Autodesk Inventor part; units mm, degrees
ref_plane "YZ Plane" through (0, 0, 0) normal (1, 0, 0) x (0, 1, 0)
ref_plane "XZ Plane" through (0, 0, 0) normal (0, 1, 0) x (-1, 0, 0)
ref_plane "XY Plane" through (0, 0, 0) normal (0, 0, 1) x (1, 0, 0)
sketch "Sketch1" plane through (0, 0, 0) normal (1, 0, 0) x (0, 1, 0)
  line L0 (0, 0) -> (4.7625, 0)
  line L1 (4.7625, 0) -> (4.7625, -168.8592)
  line L2 (4.7625, -168.8592) -> (0, -168.8592)
  line L3 (0, -168.8592) -> (0, 0)
  dimension "d1" = 4.7625
  dimension "d2" = 168.8592
extrude "Extrusion1" add sketch "Sketch1" along normal blind 0.7937
sketch "Sketch2" plane through (0, 0, -168.8592) normal (0, 0, -1) x (-1, 0, 0)
  line L0 (-0.7937, 0) -> (-0.7937, 4.7625)
  line L1 (-0.7937, 0) -> (36.0362, 0)
  line L2 (36.0362, 0) -> (36.0362, 4.7625)
  line L3 (36.0362, 4.7625) -> (-0.7937, 4.7625)
  line L4 (-0.7937, 4.7625) -> (-0.7937, 0)
  point P0 (0, 0)
  dimension "d5" = 36.83
  dimension "d6" = 4.7625
extrude "Extrusion2" add sketch "Sketch2" against normal blind 0.7937
sketch "Sketch3" plane through (-36.0362, 0, -168.8592) normal (-1, 0, 0) x (0, 0, 1)
  line L0 (168.8592, 4.7625) -> (168.8592, 0)
  line L1 (0, 0) -> (168.8592, 0)
  line L2 (168.8592, 0) -> (168.8592, 4.7625)
  line L3 (168.8592, 4.7625) -> (0, 4.7625)
  line L4 (0, 4.7625) -> (0, 0)
extrude "Extrusion3" add sketch "Sketch3" against normal blind 0.7937
sketch "Sketch4" plane through (-36.0362, 0, 0) normal (0, 0, 1) x (1, 0, 0)
  line L0 (0, 0) -> (0, 4.7625)
  line L1 (36.0362, 4.7625) -> (36.83, 4.7625)
  line L2 (0, 0) -> (36.83, 0)
  line L3 (36.83, 0) -> (36.83, 4.7625)
  line L4 (36.83, 4.7625) -> (0, 4.7625)
  line L5 (0, 4.7625) -> (0, 0)
  point P0 (36.0362, 0)
extrude "Extrusion4" add sketch "Sketch4" against normal blind 0.7937
sketch "Sketch7" plane through (-36.0362, 0, 0) normal (0, 0, 1) x (1, 0, 0)
  circle A0 centre (18.415, 2.3812) radius 2.2098
extrude "Extrusion5" cut sketch "Sketch7" against normal blind 0.7937
sketch "Sketch6" plane through (0.7937, 0, -168.8592) normal (0, 0, -1) x (-1, 0, 0)
  circle A0 centre (18.415, 2.3812) radius 2.2098
extrude "Extrusion6" cut sketch "Sketch6" against normal blind 0.7937
properties part number "Back rubber bands"
The listing builds one solid part. Answer for the finished solid, in the listing's coordinates (mm). A direction names the side the tool comes from. Give positions to 0.01 mm unless a question says otherwise; leave off trailing zeros. Write each loop counter-clockwise with the first axis right and the second up, starting at its lowest first coordinate (ties: lowest second). Pieces come first, ordered by that corner, then holes. Notation, with made-up numbers: (31.5, 23.25) -> (36.5, 23.25) arc R25 ccw to (36.5, 50.25) -> close; hole circle Ø4 at (89, 39.5). An arc over 180 degrees is marked (long way). Write item = value, one per line. Start each with the question number.
1) The part is cut by section B-B, the plane x = -13. Determine the outline of the cut face in (y, z).
2) Which of the six approach directions +Z, -Z, +X, -X, +Y, -Y give full straight-line access (tool end or side, diameter ignored) to faces 5 (the face through (0, 2, -83)), 6 (the face through (-35.4, 4.762, -84))?
3) Determine the mould class of faces 1 (the face through (-14, 2, 0)), 2 (the face through (0.794, 2, -84)), 3 (the face through (-36.036, 2, -86)), 4 (the face through (-19.83, 2.48, -0.39)) for opening direction X: +X half, -X half, draft (parallel to the pull), parting line (faces both ways), or undercut.
4) Straight lines are drawn through the part: line 1 along X through (y, z) = (4, -52.5); line 2 along Z through (x, y) = (-5, 3.75). For each, find the intervals that lie inside material, in ascending order.
5) The part is cut by section A-A, the plane z = -86. Determine the outline of the cut face in (x, y).
Solutions:
q1.outline = (0, -168.86) -> (4.76, -168.86) -> (4.76, -168.07) -> (0, -168.07) -> close; (0, -0.79) -> (4.76, -0.79) -> (4.76, 0) -> (0, 0) -> close
q2.face_5 = +Y, -Y
q2.face_6 = +Z, -Z, +X, -X, +Y
q3.face_1 = draft
q3.face_2 = +X half
q3.face_3 = -X half
q3.face_4 = undercut
q4.line_1 = -36.04 to -35.24, 0 to 0.79
q4.line_2 = -168.86 to -168.07, -0.79 to 0
q5.outline = (-36.04, 0) -> (-35.24, 0) -> (-35.24, 4.76) -> (-36.04, 4.76) -> close; (0, 0) -> (0.79, 0) -> (0.79, 4.76) -> (0, 4.76) -> close
